Here's how the part is built. I have some questions about the finished solid (model axes, mm). A direction names the side the tool comes from. Coordinates: 2 decimals unless noted, no trailing zeros. Answer as CSV lines item,"result". Start each with the question number.
Q1. For faces 4 (the face through (-2.82, 0.708, 4.93)), 5 (the face through (0.9, 1.6, 4.9)), 6 (the face through (2.009, -2.074, 4.93)), 7 (the face through (-1, -1, 10)), which set-ups out of +Z, -Z, +X, -X, +Y, -Y let a thin tool reach every point of the face, with its end or its side?
Q2. For pin 1 Ø6 at (x, z) = (3.5, 7) entering from -Y; pin 2 Ø4 at (y, z) = (2, 4) entering from -X; pin 3 Ø1 at (y, z) = (-1.5, 3.5) entering from +X, each with a flat end and sliding along its axis, tell me the tip position at first contact or that it passes through.
Q3. I need wall thicknesses on line 1 (Y direction, x = -3.25, z = 0.5); line 2 (Y direction, x = -3.75, z = 2.5); line 3 (X direction, y = -1.75, z = 2.5). Which ranges of each line are inside material? Lowest first, please.
Q4. Thinking about a two-plate mould opening in Y: for faces 1 (the face through (2.023, 2.089, 4.93)), 2 (the face through (-1, -1, 0)), 3 (the face through (-2.8, -0.703, 4.93)), which applies, released by +Y, released by -Y, zero draft, split by the parting line, or undercut?
from build123d import *

# Parameters (mm, degrees)
PAD_DEPTH = 10


with BuildPart() as part:
    # InvoluteGear → Pad (new body)
    with BuildSketch(Plane.XY):
        with BuildLine():
            Line((1.489546, -1.550404), (2.542216, -2.612039))
            add(Edge.make_bspline(
                [(2.542216, -2.612039), (2.745429, -2.736985), (3.330232, -2.991658), (4.656223, -2.658727)],
                knots=[0, 0, 0, 0, 1, 1, 1, 1], degree=3))
            add(Edge.make_bspline(
                [(4.656223, -2.658727), (6.060271, -2.106027), (7.683483, -0.764768), (8.344372, 2.4318)],
                knots=[0, 0, 0, 0, 1, 1, 1, 1], degree=3))
            add(Edge.make_bspline(
                [(8.344372, 2.4318), (7.683483, 0.764768), (6.060271, 2.106027), (4.656223, 2.658727)],
                knots=[0, 0, 0, 0, 1, 1, 1, 1], degree=3))
            add(Edge.make_bspline(
                [(4.656223, 2.658727), (3.330232, 2.991658), (2.745429, 2.736985), (2.542216, 2.612039)],
                knots=[0, 0, 0, 0, 1, 1, 1, 1], degree=3))
            Line((2.542216, 2.612039), (1.489546, 1.550404))
            ThreePointArc((1.489546, 1.550404), (0.917161, 1.58857), (0.597916, 2.065187))
            Line((0.597916, 2.065187), (0.990984, 3.507643))
            add(Edge.make_bspline(
                [(0.990984, 3.507643), (0.997584, 3.746104), (0.925736, 4.379895), (-0.025587, 5.361771)],
                knots=[0, 0, 0, 0, 1, 1, 1, 1], degree=3))
            add(Edge.make_bspline(
                [(-0.025587, 5.361771), (-1.206262, 6.301362), (-3.179433, 7.036476), (-6.278187, 6.010538)],
                knots=[0, 0, 0, 0, 1, 1, 1, 1], degree=3))
            add(Edge.make_bspline(
                [(-6.278187, 6.010538), (-4.50405, 6.271708), (-4.854008, 4.195335), (-4.630636, 2.703044)],
                knots=[0, 0, 0, 0, 1, 1, 1, 1], degree=3))
            add(Edge.make_bspline(
                [(-4.630636, 2.703044), (-4.255968, 1.388236), (-3.743013, 1.009119), (-3.5332, 0.895604)],
                knots=[0, 0, 0, 0, 1, 1, 1, 1], degree=3))
            Line((-3.5332, 0.895604), (-2.087462, 0.514783))
            ThreePointArc((-2.087462, 0.514783), (-1.834323, 0), (-2.087462, -0.514783))
            Line((-2.087462, -0.514783), (-3.5332, -0.895604))
            add(Edge.make_bspline(
                [(-3.5332, -0.895604), (-3.743013, -1.009119), (-4.255968, -1.388236), (-4.630636, -2.703044)],
                knots=[0, 0, 0, 0, 1, 1, 1, 1], degree=3))
            add(Edge.make_bspline(
                [(-4.630636, -2.703044), (-4.854008, -4.195335), (-4.50405, -6.271708), (-2.066185, -8.442338)],
                knots=[0, 0, 0, 0, 1, 1, 1, 1], degree=3))
            add(Edge.make_bspline(
                [(-2.066185, -8.442338), (-3.179433, -7.036476), (-1.206262, -6.301362), (-0.025587, -5.361771)],
                knots=[0, 0, 0, 0, 1, 1, 1, 1], degree=3))
            add(Edge.make_bspline(
                [(-0.025587, -5.361771), (0.925736, -4.379895), (0.997584, -3.746104), (0.990984, -3.507643)],
                knots=[0, 0, 0, 0, 1, 1, 1, 1], degree=3))
            Line((0.990984, -3.507643), (0.597916, -2.065187))
            ThreePointArc((0.597916, -2.065187), (0.917161, -1.58857), (1.489546, -1.550404))
        make_face()
    extrude(amount=PAD_DEPTH)


solid = part.part
Here are the results:
1,face 4,"+Z, -Z, -X"
1,face 5,"+Z, -Z"
1,face 6,"+Z, -Z, -Y"
1,face 7,"+Z, +X, -X, +Y, -Y"
2,pin 1,"stops at y = -4.74"
2,pin 2,"stops at x = -4.74"
2,pin 3,"stops at x = 6.86"
3,line 1,"y = -7.21 to -0.82, 0.82 to 6.5"
3,line 2,"y = -6.51 to -1.05, 1.05 to 6.5"
3,line 3,"x = -4.27 to 0.73, 1.69 to 6.15"
4,face 1,"released by +Y"
4,face 2,"zero draft"
4,face 3,"undercut"
